```python
from build123d import *

# Parameters (mm, degrees)
SKETCH1_R          = 10
SKETCH1_R_2        = 8
EXTRUDE1_DEPTH     = 17
EXTRUDE3_START     = -9
SKETCH2_R          = 8
EXTRUDE3_DEPTH     = 10.5
SKETCH3_R          = 10.5
EXTRUDE4_DEPTH     = 1
SKETCH4_R          = 4.5
CUT_EXTRUDE1_DEPTH = 5
SKETCH6_R          = 2
CUT_EXTRUDE4_DEPTH = 5
CIRPATTERN1_COUNT  = 4
SKETCH7_W          = 0.4
SKETCH7_H          = 0.4
CUT_EXTRUDE5_DEPTH = 14.5
CIRPATTERN2_COUNT  = 4


with BuildPart() as part:
    # Sketch1 → Extrude1 (new body)
    with BuildSketch(Plane(origin=(0, 0, 0), x_dir=(1, 0, 0), z_dir=(0, 1, 0))):
        Circle(SKETCH1_R)
        Circle(SKETCH1_R_2, mode=Mode.SUBTRACT)
    extrude(amount=EXTRUDE1_DEPTH)

    # Sketch2 → Extrude3 (add)
    with BuildSketch(Plane(origin=(0, 17, 0), x_dir=(-1, 0, 0), z_dir=(0, 1, 0)).offset(EXTRUDE3_START)):
        Circle(SKETCH2_R)
    extrude(amount=EXTRUDE3_DEPTH)

    # Sketch3 → Extrude4 (add)
    with BuildSketch(Plane(origin=(0, 17, 0), x_dir=(-1, 0, 0), z_dir=(0, 1, 0))):
        Circle(SKETCH3_R)
    extrude(amount=EXTRUDE4_DEPTH)

    # Sketch4 → Cut-Extrude1 (cut)
    with BuildSketch(Plane(origin=(0, 18.5, 0), x_dir=(-1, 0, 0), z_dir=(0, 1, 0))):
        Circle(SKETCH4_R)
    extrude(amount=-CUT_EXTRUDE1_DEPTH, mode=Mode.SUBTRACT)

    # Sketch6 → Cut-Extrude4 (cut)
    with BuildSketch(Plane.XZ.offset(-8)):
        with Locations((6, 0)):
            Circle(SKETCH6_R)
    cut_extrude4 = extrude(amount=-CUT_EXTRUDE4_DEPTH, mode=Mode.SUBTRACT)

    # CirPattern1: Cut-Extrude4 ×4 about axis
    cirpattern1_axis = Axis((0, 0, 0), (0, 1, 0))
    for i in range(1, CIRPATTERN1_COUNT):
        add(cut_extrude4.rotate(cirpattern1_axis, i * 360 / CIRPATTERN1_COUNT), mode=Mode.SUBTRACT)

    # Sketch7 → Cut-Extrude5 (cut, through all)
    with BuildSketch(Plane(origin=(0, 13.5, 0), x_dir=(-1, 0, 0), z_dir=(0, 1, 0))):
        with Locations((-4.259587971, 0)):
            Rectangle(SKETCH7_W, SKETCH7_H)
    cut_extrude5 = extrude(amount=-CUT_EXTRUDE5_DEPTH, mode=Mode.SUBTRACT)

    # CirPattern2: Cut-Extrude5 ×4 about axis
    cirpattern2_axis = Axis((0, 0, 0), (0, 1, 0))
    for i in range(1, CIRPATTERN2_COUNT):
        add(cut_extrude5.rotate(cirpattern2_axis, i * 360 / CIRPATTERN2_COUNT), mode=Mode.SUBTRACT)


solid = part.part
```
Input: part model. Units: mm. Frame: model coordinates. A direction names the side the tool comes from. Coordinates: 2 decimals unless noted, no trailing zeros. Write each loop counter-clockwise with the first axis right and the second up, starting at its lowest first coordinate (ties: lowest second). Pieces come first, ordered by that corner, then holes.
1) Section D-D on x = 6. Output: boundary loops of the cut face in (y, z), and give its area (3 significant figures).
2) Section B-B on x = -2.75. Output: boundary loops of the cut face in (y, z), and give its area (3 significant figures).
3) Pin query (flat end, axial travel): pin 1 Ø3 at (y, z) = (14.5, -1) entering from -X; pin 2 Ø3 at (x, y) = (5.5, 16.5) entering from -Z; pin 3 Ø2 at (x, z) = (-6, 0) entering from -Y. Return the tip coordinate at first contact, or that it passes through.
4) Section C-C on z = -1.25. Output: boundary loops of the cut face in (x, y), and give its area (3 significant figures).
5) Section A-A on y = 15.25. Output: boundary loops of the cut face in (x, z), and give its area (3 significant figures).
6) Set-up query: faces 1 (the flat face through (2, 18, -8)), 2 (the flat face through (0, 8, 0)), 3 (the flat face through (-3.4, 18.5, -3.4)). Return all of +Z, -Z, +X, -X, +Y, -Y with unobstructed straight access to the full face (end or side cutting, diameter ignored); none if empty.
7) Mould query, pull axis X, two halves, no side actions, for faces 4 (the flat face through (0, 0, -8.2)), 5 (the flat face through (-6, 13, 0)), 6 (the flat face through (0, 13.5, 0)), 7 (the cylindrical face through (-10, 17.5, 3.2)). Classes: pulls with the +X half, pulls with the -X half, needs draft (parallel to the pull), parting line crosses it, or undercut.
8) Material intervals for line 1 along X through (y, z) = (2.5, 0); line 2 along Z through (x, y) = (0, 15); line 3 along Z through (x, y) = (-1.25, 8.5), sorted ascending.
Check result:
1. outline: (0, -8) - (17, -8) - (17, -8.62) - (18, -8.62) - (18, -5.29) - (18.5, -5.29) - (18.5, 5.29) - (18, 5.29) - (18, 8.62) - (17, 8.62) - (17, 8) - (0, 8) - (0, 5.29) - (8, 5.29) - (8, 2) - (13, 2) - (13, -2) - (8, -2) - (8, -5.29) - (0, -5.29) - close
1. area: 190 mm2
2. outline: (0, -9.61) - (17, -9.61) - (17, -10.13) - (18, -10.13) - (18, -7.51) - (18.5, -7.51) - (18.5, -3.56) - (13.5, -3.56) - (13.5, 3.56) - (18.5, 3.56) - (18.5, 7.51) - (18, 7.51) - (18, 10.13) - (17, 10.13) - (17, 9.61) - (0, 9.61) - (0, 7.51) - (8, 7.51) - (8, -7.51) - (0, -7.51) - close
2. area: 199 mm2
3. pin 1: stops at x = -10
3. pin 2: stops at z = -9.67
3. pin 3: stops at y = 13
4. outline: (-10.43, 17) - (-9.92, 17) - (-9.92, 0) - (-7.9, 0) - (-7.9, 8) - (-7.56, 8) - (-7.56, 13) - (-4.44, 13) - (-4.44, 8) - (4.44, 8) - (4.44, 13) - (7.56, 13) - (7.56, 8) - (7.9, 8) - (7.9, 0) - (9.92, 0) - (9.92, 17) - (10.43, 17) - (10.43, 18) - (7.9, 18) - (7.9, 18.5) - (4.32, 18.5) - (4.32, 13.5) - (-4.32, 13.5) - (-4.32, 18.5) - (-7.9, 18.5) - (-7.9, 18) - (-10.43, 18) - close
4. area: 165 mm2
5. outline: circle Ø20 at (0, 0); hole circle Ø9 at (0, 0)
5. area: 251 mm2
6. face 1: +Y
6. face 2: -Y
6. face 3: +Z, -Z, +X, -X, +Y
7. face 4: needs draft
7. face 5: undercut
7. face 6: undercut
7. face 7: parting line crosses it
8. line 1: x = -10 to -8, 8 to 10
8. line 2: z = -10 to -4.5, 4.5 to 10
8. line 3: z = -9.92 to -7.56, -4.44 to 4.44, 7.56 to 9.92
